Part print with two shaded views. Sizes in mm from the minimum x, y, z corner. Give positions to 0.01 mm unless a question says otherwise; leave off trailing zeros. Write each loop counter-clockwise with the first axis right and the second up, starting at its lowest first coordinate (ties: lowest second). Pieces come first, ordered by that corner, then holes. Notation, with made-up numbers: (23, 11.5) - (32, 11.5) arc R29 cw to (32, 41.5) - close; hole circle Ø5 at (89.25, 61.25). An arc over 180 degrees is marked (long way). One line per item, written item: value. Start each with the question number.
(1) Drop flat-ended pins along their axis: P1, Ø12, axis at x = 7, z = 85, coming from the +Y side; P2, Ø10, axis at y = 469.5, z = 226, coming from the -X side; P3, Ø1, axis at x = 8.5, z = 414, coming from the +Y side. Give the stop position or say it passes through.
(2) Cut at B-B, the plane y = 603. List the corners of the cut face in (x, z).
(3) Cut at A-A, the plane z = 250. List the corners of the cut face in (x, y).
(4) Mould opens along X. For the marked faces 1 and 2 say: pulls with the +X half, pulls with the -X half, needs draft (parallel to the pull), parting line crosses it, or undercut.
(5) Cut at C-C, the plane z = 80. List the corners of the cut face in (x, y).
(6) Probe L1, parallel to Z at x = 59.25, y = 1453; L2, parallel to Z at x = 42.75, y = 1453; L3, parallel to X at y = 842.5, z = 331.5. List the from-to ranges inside material, lowest first.
(7) Cut at D-D, the plane z = 333. List the corners of the cut face in (x, y), and give its area (3 significant figures).
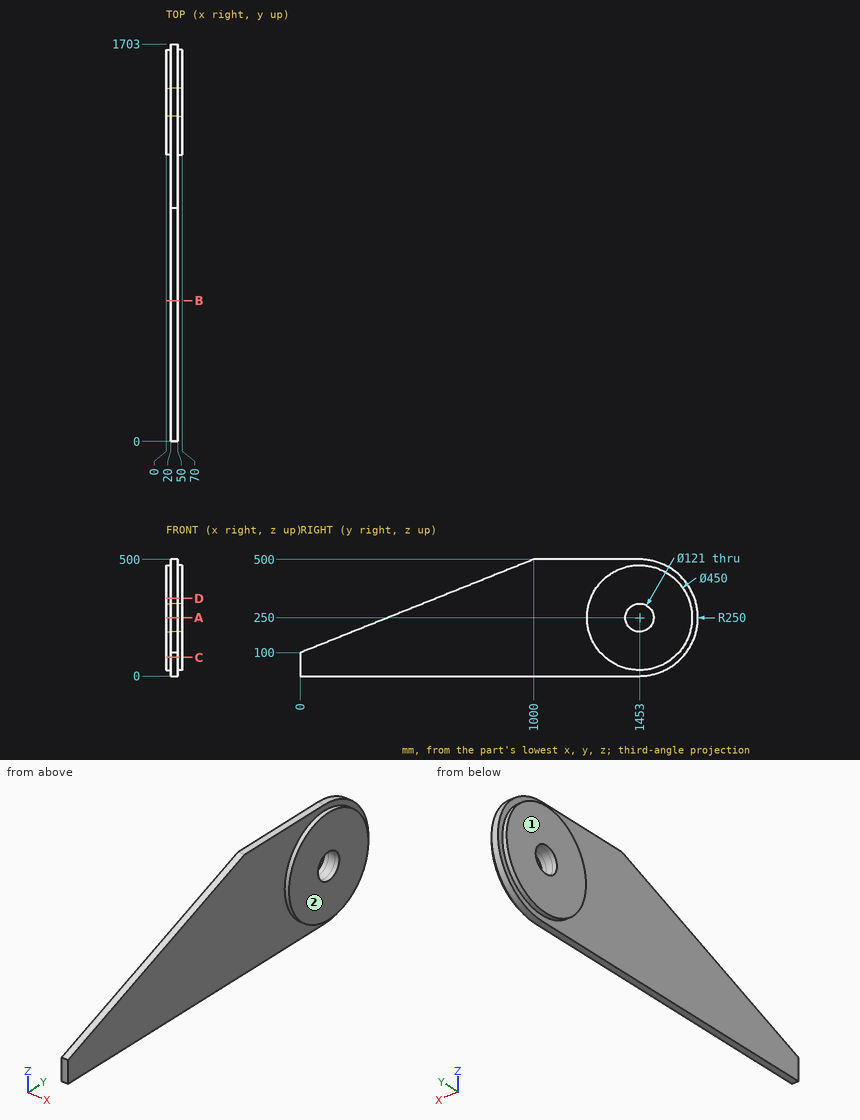
Answers follow:
1. P1: stops at y = 1612.2
1. P2: stops at x = 20
1. P3: stops at y = 1607.57
2. outline: (20, 0) - (50, 0) - (50, 341.2) - (20, 341.2) - close
3. outline: (0, 1228) - (20, 1228) - (20, 375) - (50, 375) - (50, 1228) - (70, 1228) - (70, 1392.5) - (0, 1392.5) - close; (0, 1513.5) - (70, 1513.5) - (70, 1678) - (50, 1678) - (50, 1703) - (20, 1703) - (20, 1678) - (0, 1678) - close
4. face 1: pulls with the -X half
4. face 2: pulls with the +X half
5. outline: (0, 1305.61) - (20, 1305.61) - (20, 0) - (50, 0) - (50, 1305.61) - (70, 1305.61) - (70, 1600.39) - (50, 1600.39) - (50, 1636.3) - (20, 1636.3) - (20, 1600.39) - (0, 1600.39) - close
6. L1: z = 25 to 189.5, 310.5 to 475
6. L2: z = 0 to 189.5, 310.5 to 500
6. L3: x = 20 to 50
7. outline: (0, 1243.87) - (20, 1243.87) - (20, 582.5) - (50, 582.5) - (50, 1243.87) - (70, 1243.87) - (70, 1662.13) - (50, 1662.13) - (50, 1688.82) - (20, 1688.82) - (20, 1662.13) - (0, 1662.13) - close
7. area: 49,900 mm²
